```python
from build123d import *

# Parameters (mm, degrees)
F0_R            = 50
F1_DEPTH        = 40
F2_D            = 12.1
F3_SIZE         = 5
F4_DEPTH        = 300
F6_DEPTH        = 25
F7_SIZE         = 10
F8_R            = 10
F10_D           = 17.5
F10_CBORE_D     = 31.5
F10_CBORE_DEPTH = 20


with BuildPart() as f1:
    # F0 (on Front) → F1 (new body)
    with BuildSketch(Plane.XZ):
        Polygon((-100, 0), (0, 0), (100, 0), (100, 40), (-100, 40), align=None)
        with BuildLine():
            Line((-100, 40), (100, 40))
            Line((100, 40), (100, 200))
            ThreePointArc((100, 200), (0, 100), (-100, 200))
            Line((-100, 200), (-100, 40))
        make_face()
        with BuildLine():
            ThreePointArc((-100, 200), (0, 100), (100, 200))
            ThreePointArc((100, 200), (0, 300), (-100, 200))
        make_face()
        with Locations((0, 200)):
            Circle(F0_R, mode=Mode.SUBTRACT)
    extrude(amount=F1_DEPTH)

    # F2 (through all)
    with Locations(Plane(origin=(0, 0, 0), x_dir=(1, 0, 0), z_dir=(0, 1, 0))):
        with Locations((72, -200), (0, -128), (-72, -200), (0, -272)):
            Hole(F2_D / 2)

    # F3
    f3_edges = [f1.edges().sort_by_distance(p)[0] for p in [
        (-100, -20, 0),
        (100, -20, 0),
    ]]
    chamfer(f3_edges, length=F3_SIZE)

    # F0 (on Front) → F4 (join)
    with BuildSketch(Plane.XZ):
        Polygon((-100, 0), (0, 0), (100, 0), (100, 40), (-100, 40), align=None)
    extrude(amount=F4_DEPTH)

    # F5 (on Right) → F6 (join, symmetric)
    with BuildSketch(Plane.YZ):
        Polygon((-100, 40), (-40, 40), (-40, 100), align=None)
    extrude(amount=F6_DEPTH, both=True)

    # F7
    f7_edges = [f1.edges().sort_by_distance(p)[0] for p in [
        (-100, -300, 20),
        (100, -300, 20),
        (0, 0, 0),
    ]]
    chamfer(f7_edges, length=F7_SIZE)

    # F8
    f8_edges = [f1.edges().sort_by_distance(p)[0] for p in [
        (-62.5, -40, 40),
        (62.5, -40, 40),
    ]]
    fillet(f8_edges, radius=F8_R)

    # F10 (through all)
    with Locations(Plane.XY.offset(40)):
        with Locations((60, -140), (60, -260), (-60, -260), (-60, -140)):
            CounterBoreHole(F10_D / 2, F10_CBORE_D / 2, F10_CBORE_DEPTH)


solid = f1.part
```
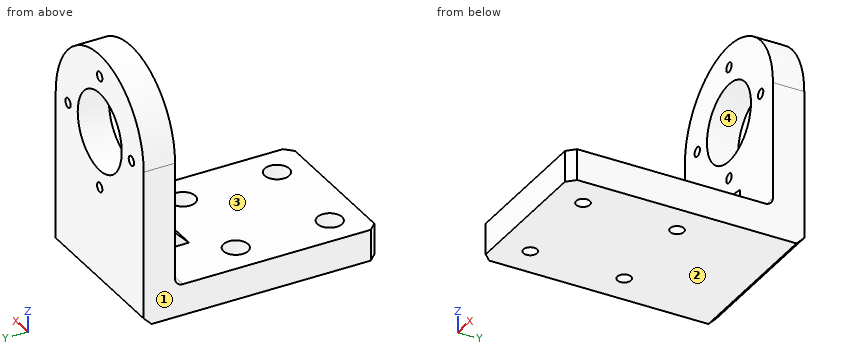
Design review of the part built by this model. Coordinates are the model's own, in mm. Face numbers are marked on the shaded views. Coordinates: 2 decimals unless noted, no trailing zeros. Order: outer loops, then holes, each group sorted by start corner. A loop starts at its lowest first (then second) coordinate and runs counter-clockwise, first axis right, second up. Notation, with made-up numbers: M -39.5,-11.75 L -2.5,-11.75 A11 ccw -2.5,6.25 Z; hole C -28.75,27.25 d2. An arc over 180 degrees is marked long. Answer as a JSON object with one key per item and string values. Group by question number.
1) Add section B-B, the plane z = 128. Write out the cut boundary in (x, y), then the cut area to 3 significant figures.
2) Mouldability with a two-part tool opening along Z and no side actions: class the marked faces 1, 2, 3 and 4 as pulls with the +Z half, pulls with the -Z half, needs draft (parallel to the pull), parting line crosses it, or undercut.
3) Add section D-D, the plane x = 0. Write out the cut boundary in (y, z).
4) For pin 1 (19.5 mm diameter, centred on x = 0, z = 128, fed in from -Y); pin 2 (25 mm diameter, centred on x = 57, y = -267.5, fed in from +Z); pin 3 (16 mm diameter, centred on x = -65.5, y = -255, fed in from +Z); pin 4 (14 mm diameter, centred on x = 60, y = -260, fed in from -Z), all flat-tipped, find the tip position at first contact; note any pin that passes through.
5) Add section A-A, the plane x = -60. Write out the cut boundary in (y, z).
6) Add section C-C, the plane y = -140. Write out the cut boundary in (x, z).
7) Wall thickness on L1, parallel to X at y = -29, z = 128; L2, parallel to Z at x = 0, y = -20; L3, parallel to Y at x = 60, z = 7.25: over which ranges is each line inside the solid? List them lowest first.
Computed values:
{
 "1": {"outline": "M -100,-40 L -6.05,-40 L -6.05,0 L -100,0 Z; M 6.05,-40 L 100,-40 L 100,0 L 6.05,0 Z", "area": "7,520 mm^2"},
 "2": {"face 1": "needs draft", "face 2": "pulls with the -Z half", "face 3": "pulls with the +Z half", "face 4": "undercut"},
 "3": {"outline": "M -300,0 L -10,0 L 0,10 L 0,121.95 L -40,121.95 L -40,100 L -100,40 L -300,40 Z; M -40,134.05 L 0,134.05 L 0,150 L -40,150 Z; M -40,250 L 0,250 L 0,265.95 L -40,265.95 Z; M -40,278.05 L 0,278.05 L 0,300 L -40,300 Z"},
 "4": {"pin 1": "stops at y = -40", "pin 2": "stops at z = 40", "pin 3": "stops at z = 20", "pin 4": "passes through"},
 "5": {"outline": "M -300,0 L -268.75,0 L -268.75,20 L -275.75,20 L -275.75,40 L -300,40 Z; M -251.25,0 L -148.75,0 L -148.75,20 L -155.75,20 L -155.75,40 L -244.25,40 L -244.25,20 L -251.25,20 Z; M -131.25,0 L -10,0 L 0,10 L 0,280 L -40,280 L -40,50 A10 cw -50,40 L -124.25,40 L -124.25,20 L -131.25,20 Z"},
 "6": {"outline": "M -100,0 L -68.75,0 L -68.75,20 L -75.75,20 L -75.75,40 L -100,40 Z; M -51.25,0 L 51.25,0 L 51.25,20 L 44.25,20 L 44.25,40 L -44.25,40 L -44.25,20 L -51.25,20 Z; M 68.75,0 L 100,0 L 100,40 L 75.75,40 L 75.75,20 L 68.75,20 Z"},
 "7": {"L1": "x = -100 to -6.05, 6.05 to 100", "L2": "z = 0 to 121.95, 134.05 to 150, 250 to 265.95, 278.05 to 300", "L3": "y = -300 to -268.75, -251.25 to -148.75, -131.25 to -2.75"}
}
